Read the model definition and answer for the solid it produces. Units are mm, in the model's axes. A direction names the side the tool comes from. Give positions to 0.01 mm unless a question says otherwise; leave off trailing zeros. Write each loop counter-clockwise with the first axis right and the second up, starting at its lowest first coordinate (ties: lowest second). Pieces come first, ordered by that corner, then holes. Notation, with made-up numbers: M 20,-25 L 62,-25 A22 ccw 62,-13 Z; hole C -39,54 d1. An arc over 180 degrees is marked long. Use a Markdown table: item, result. Add a question column.
Item 1: A cutting plane is placed at A-A on z = 2.5. Determine the outline of the cut face in (x, y).
Item 2: Given P1, Ø2, axis at x = 4, z = 3, coming from the +Y side; P2, Ø2.5, axis at x = -18, y = -12.5, coming from the +Z side; P3, Ø3.5, axis at y = -7.5, z = 7, coming from the +X side, each flat-ended and moving along its own axis, determine where each tip first touches the part or whether it passes through.
Item 3: A cutting plane is placed at D-D on z = 7.5. Determine the outline of the cut face in (x, y), then the cut area to 3 significant figures.
Item 4: The mould has two halves that part along Y. Classify faces 1 (the flat face through (0, -18.3, 6)), 2 (the cylindrical face through (0.1, -5.5, 5.5)), 3 (the flat face through (-4, -13.5, 2)), 4 (the cylindrical face through (0, -3, 5)): pulls with the +Y half, pulls with the -Y half, needs draft (parallel to the pull), parting line crosses it, or undercut.
Item 5: For faces 5 (the flat face through (3, -16, 2)), 6 (the flat face through (-16.25, -9, 7)), 7 (the flat face through (18, -9, 5)), 8 (the flat face through (-4, -6, 2)), determine the directions among +Z, -Z, +X, -X, +Y, -Y from which every point of the face is accessible in a straight line to the end or side of a thin tool.
Item 6: A cutting plane is placed at C-C on x = 0. Determine the outline of the cut face in (y, z), then the cut area to 3 significant figures.
Item 7: A cutting plane is placed at B-B on y = -5.5. Determine the outline of the cut face in (x, z).
Item 8: Consider probe 1 along X at (y, z) = (-2.4, 2.5); probe 2 along X at (y, z) = (-9, 3); probe 3 along Y at (x, z) = (3.5, 2.25). Determine where each line is inside the solid, lowest interval first. Write a range as [from, to].
from build123d import *

# Parameters (mm, degrees)
PAD_DEPTH       = 18.3
POCKET_DEPTH    = 5
SKETCH004_W     = 5
SKETCH004_H     = 6
POCKET001_DEPTH = 2


with BuildPart() as part:
    # Sketch → Pad (new body)
    with BuildSketch(Plane.XZ):
        Polygon((-19.25, 0), (19.25, 0), (19.25, 5), (16.25, 5), (16.25, 8), (-16.25, 8), (-16.25, 5), (-19.25, 5), align=None)
    extrude(amount=PAD_DEPTH)

    # Sketch001 (on Face1 of Pad) → Pocket (cut)
    with BuildSketch(Plane(origin=(0, 0, 0), x_dir=(1, 0, 0), z_dir=(0, 0, -1))):
        Polygon((4.25, 13.5), (4.25, 6), (-4.25, 6), (-4.25, 13.5), (-3, 13.5), (-3, 18.5), (3, 18.5), (3, 13.5), align=None)
    extrude(amount=-POCKET_DEPTH, mode=Mode.SUBTRACT)

    # Sketch003 → Groove (revolve, cut)
    with BuildSketch(Plane.YZ):
        Polygon((0, 2.5), (0, 5), (-5, 5), (-5, 5.5), (-6, 5.5), (-6, 2.5), align=None)
    revolve(axis=Axis((0, 0, 2.5), (0, -1, 0)), mode=Mode.SUBTRACT)

    # Sketch004 (on Face1 of Groove) → Pocket001 (cut)
    with BuildSketch(Plane(origin=(0, 0, 0), x_dir=(1, 0, 0), z_dir=(0, 0, -1))):
        with Locations((0, 3)):
            Rectangle(SKETCH004_W, SKETCH004_H)
    extrude(amount=-POCKET001_DEPTH, mode=Mode.SUBTRACT)


solid = part.part
Filled in:
| question | item | result |
|---|---|---|
| 1 | outline | M -19.25,-18.3 L -3,-18.3 L -3,-13.5 L -4.25,-13.5 L -4.25,-6 L -3,-6 L -3,-5 L -2.5,-5 L -2.5,0 L -19.25,0 Z; M 2.5,-5 L 3,-5 L 3,-6 L 4.25,-6 L 4.25,-13.5 L 3,-13.5 L 3,-18.3 L 19.25,-18.3 L 19.25,0 L 2.5,0 Z |
| 2 | P1 | y = 0 |
| 2 | P2 | z = 5 |
| 2 | P3 | x = 16.25 |
| 3 | outline | M -16.25,-18.3 L 16.25,-18.3 L 16.25,0 L -16.25,0 Z |
| 3 | area | 595 mm² |
| 4 | face 1 | pulls with the -Y half |
| 4 | face 2 | undercut |
| 4 | face 3 | undercut |
| 4 | face 4 | needs draft |
| 5 | face 5 | -Z, -Y |
| 5 | face 6 | +Z, -X, +Y, -Y |
| 5 | face 7 | +Z, +X, +Y, -Y |
| 5 | face 8 | -Z |
| 6 | outline | M -18.3,5 L -6,5 L -6,5.5 L -5,5.5 L -5,5 L 0,5 L 0,8 L -18.3,8 Z |
| 6 | area | 54.4 mm² |
| 7 | outline | M -19.25,0 L -2.5,0 L -2.5,0.84 A3 cw long 2.5,0.84 L 2.5,0 L 19.25,0 L 19.25,5 L 16.25,5 L 16.25,8 L -16.25,8 L -16.25,5 L -19.25,5 Z |
| 8 | probe 1 | [-19.25, -2.5], [2.5, 19.25] |
| 8 | probe 2 | [-19.25, -4.25], [4.25, 19.25] |
| 8 | probe 3 | [-18.3, -13.5], [-6, 0] |
